Read the model definition and answer for the solid it produces. Units are mm, in the model's axes. A direction names the side the tool comes from. Round coordinates to 2 decimals unless told otherwise and drop trailing zeros. Write each loop counter-clockwise with the first axis right and the second up, starting at its lowest first coordinate (ties: lowest second). Pieces come first, ordered by that corner, then holes. Notation, with made-up numbers: (58, -33.75) -> (76, -33.75) arc R14 cw to (76, -10.75) -> close; hole circle Ø6 at (45.25, -31.75). An arc over 180 degrees is marked (long way). Return JSON: item names as keys, results as strings.
Autodesk Inventor part; units mm, degrees
ref_plane "YZ Plane" through (0, 0, 0) normal (1, 0, 0) x (0, 1, 0)
ref_plane "XZ Plane" through (0, 0, 0) normal (0, 1, 0) x (-1, 0, 0)
ref_plane "XY Plane" through (0, 0, 0) normal (0, 0, 1) x (1, 0, 0)
sketch "Sketch1" plane through (0, 0, 0) normal (0, 1, 0) x (-1, 0, 0)
  circle A0 centre (0, 0) radius 12.5
  circle A1 centre (0, 0) radius 3.1
  line L0 (-0.5, 3.0594) -> (-0.5, -3.0594)
  line L1 (0.5, -3.0594) -> (0.5, 3.0594)
  line L2 (0.5, 3.0594) -> (-0.5, -3.0594) construction
  line L3 (-0.5, 3.0594) -> (0.5, -3.0594) construction
  dimension "d0" = 6.2
  dimension "d1" = 25
  dimension "d3" = 1
extrude "Extrusion1" add sketch "Sketch1" along normal blind 7
extrude "Extrusion2" add sketch "Sketch1" along normal blind 7 contours L1 A1 L0
extrude "Extrusion3" add sketch "Sketch1" against normal blind 2 contours A0 | A1 L1 | L1 A1 L0 | L0 A1
fillet "Fillet1" radius 2 1 edges at (12.5, -2, 0)
properties part number "volumeKnob"
Item 1: For a pull along Z with two mould halves and no side action, classify faces 1 (the cylindrical face through (-11.923, 3.451, -3.755)), 2 (the flat face through (0.5, 3, 0)), 3 (the flat face through (-0.5, 3, 0)), 4 (the flat face through (0, -2, 0)) as released by +Z, released by -Z, zero draft, split by the parting line, or undercut.
Worked answers:
{"face 1": "split by the parting line", "face 2": "undercut", "face 3": "undercut", "face 4": "zero draft"}
Item 2: Section B-B (z = 0) is taken. Give the vertices of the cut face in (x, y), then the cut area to 3 significant figures.
Worked answers:
{"outline": "(-12.5, 0) arc R2 ccw to (-10.5, -2) -> (10.5, -2) arc R2 ccw to (12.5, 0) -> (12.5, 7) -> (3.1, 7) -> (3.1, 0) -> (0.5, 0) -> (0.5, 7) -> (-0.5, 7) -> (-0.5, 0) -> (-3.1, 0) -> (-3.1, 7) -> (-12.5, 7) -> close", "area": "187 mm2"}
Item 3: Straight lines are drawn through the part: L1, parallel to Y at x = -4.75, z = -9.5; L2, parallel to X at y = 6, z = 11; L3, parallel to X at y = 2, z = -3.25. For each, find the intervals that lie inside material, in ascending order. Write a range as [from, to].
Worked answers:
{"L1": "y = [-2, 7]", "L2": "x = [-5.94, 5.94]", "L3": "x = [-12.07, 12.07]"}
Item 4: Section A-A (y = 1.5) is taken. Give the vertices of the cut face in (x, z).
Worked answers:
{"outline": "circle Ø25 at (0, 0); hole (-0.5, -3.06) -> (-0.5, 3.06) arc R3.1 ccw to start; hole (0.5, -3.06) arc R3.1 ccw to (0.5, 3.06) -> close"}
Item 5: A tool of negligible diameter and unlimited length cuts with its end or side. For faces 5 (the flat face through (2, 0, 0)), 6 (the flat face through (0, 7, 0)), from which of +Z, -Z, +X, -X, +Y, -Y can it reach the whole face along a straight path? Write none if from no direction.
Worked answers:
{"face 5": "+Y", "face 6": "+Z, -Z, +X, -X, +Y"}
Item 6: Flat-ended cylindrical pins translate along their axes: pin 1 (1.5 mm diameter, centred on y = -1, z = 4.5, fed in from +X); pin 2 (1.3 mm diameter, centred on x = -2, z = -1, fed in from +Y); pin 3 (1 mm diameter, centred on x = -1.5, y = 5.5, fed in from -Z). Find the tip coordinate at first contact, or state that the pin passes through.
Worked answers:
{"pin 1": "stops at x = 11.8", "pin 2": "stops at y = 0", "pin 3": "stops at z = -12.46"}
